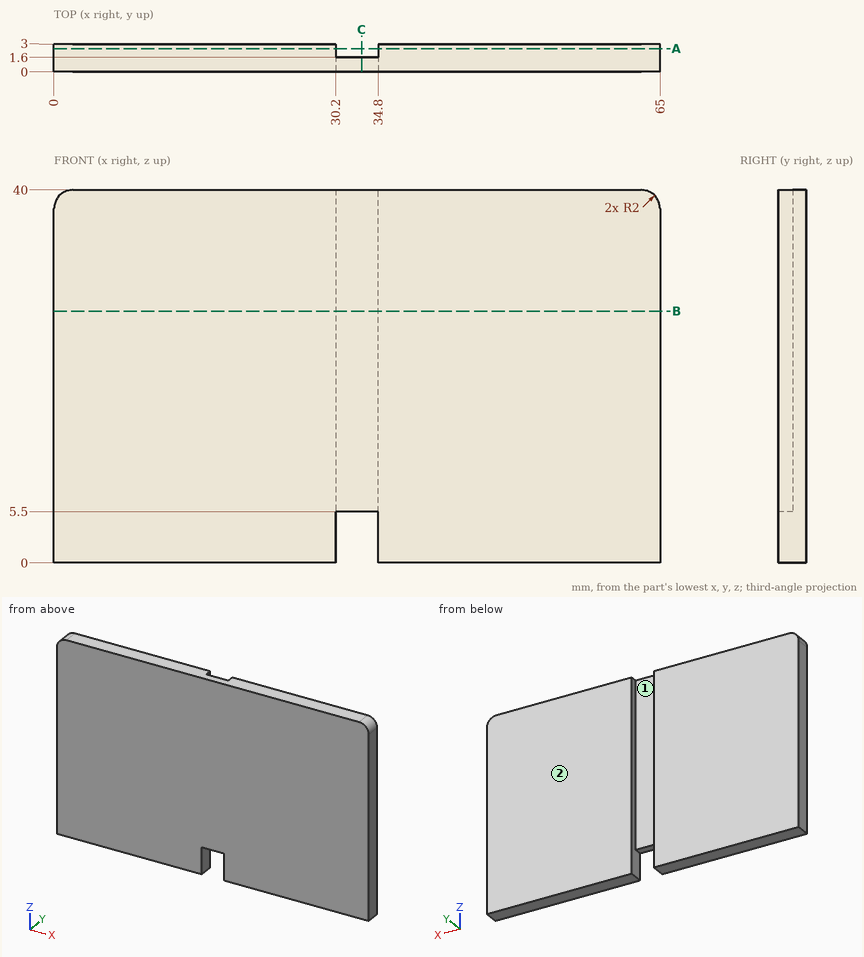
Geometry: see drawing. Coordinates: mm, zero at the bounding-box minimum. Round coordinates to 2 decimals unless told otherwise and drop trailing zeros. Order: outer loops, then holes, each group sorted by start corner. A loop starts at its lowest first (then second) coordinate and runs counter-clockwise, first axis right, second up. Notation, with made-up numbers: (-10.75, -35) - (3.25, -35) arc R20 ccw to (3.25, -3) - close; hole circle Ø6 at (7, -25). An arc over 180 degrees is marked (long way). One line per question, with ' | ' between items. Start each with the question number.
1) Cut plane B-B, the plane z = 27. Return the cut outline in (x, y), then the cut area to 3 significant figures.
2) Contact query for flat-ended pins moving along their axis: P1, Ø3.5, axis at x = 33, z = 18, coming from the +Y side; P2, Ø1.3, axis at x = 33, y = 1, coming from the -Z side. Output: stop coordinate, or through.
3) Ray query, probe 1 along X at (y, z) = (2.45, 35); probe 2 along Z at (x, y) = (34, 1.45). Return the intervals inside material, ascending.
4) Cut plane A-A, the plane y = 2.5. Return the cut outline in (x, z), then the cut area to 3 significant figures.
5) Cut plane C-C, the plane x = 33. Return the cut outline in (y, z).
6) Pull-direction query (X, two-part tool) for the marked faces 1 and 2; classes: +X half, -X half, draft (parallel to the pull), parting line (faces both ways), or undercut.
Worked out:
1) outline: (0, 0) - (65, 0) - (65, 3) - (34.8, 3) - (34.8, 1.6) - (30.2, 1.6) - (30.2, 3) - (0, 3) - close | area: 189 mm^2
2) P1: stops at y = 1.6 | P2: stops at z = 5.5
3) probe 1: x = 0 to 30.2, 34.8 to 65 | probe 2: z = 5.5 to 40
4) outline: (0, 0) - (30.2, 0) - (30.2, 40) - (2, 40) arc R2 ccw to (0, 38) - close; (34.8, 0) - (65, 0) - (65, 38) arc R2 ccw to (63, 40) - (34.8, 40) - close | area: 2,410 mm^2
5) outline: (0, 5.5) - (1.6, 5.5) - (1.6, 40) - (0, 40) - close
6) face 1: undercut | face 2: draft
